Work out the finished part from the listing and answer in its coordinate system (mm). Coordinates: 2 decimals unless noted, no trailing zeros. Loops run counter-clockwise (first coordinate to the right, second up) from the corner with the lowest first, then second, coordinate; pieces in that order, holes last. Notation, with made-up numbers: (38, 55) -> (92, 55) arc R7 cw to (92, 68) -> close; hole circle Ø6 at (-2.5, 14). An arc over 180 degrees is marked (long way). Answer as CSV lines item,"result".
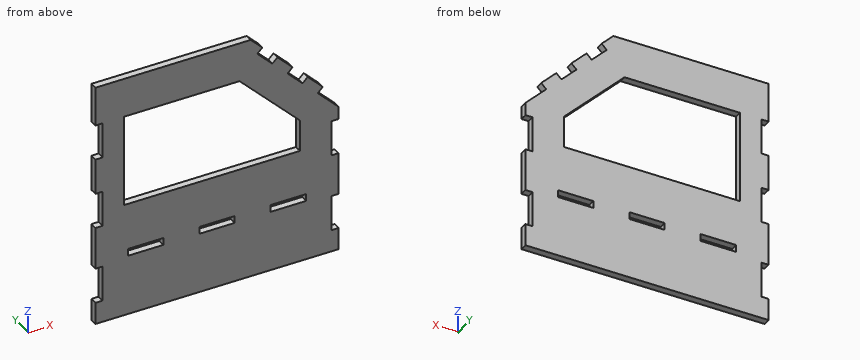
```python
from build123d import *

# Parameters (mm, degrees)
SKETCH_W  = 49.6
SKETCH_H  = 10
PAD_DEPTH = 10


with BuildPart() as part:
    # Sketch → Pad (new body)
    with BuildSketch(Plane.XZ):
        Polygon((0, 0), (0, 30.933), (10, 30.933), (10, 80.733), (0, 80.733), (0, 140.2), (10, 140.2), (10, 190), (0, 190), (0, 240), (10, 240), (10, 289.8), (0, 289.8), (0, 345), (217.0709, 345), (233.405067, 328.665833), (226.333999, 321.594766), (247.405781, 300.522983), (254.476849, 307.594051), (275.690052, 286.380848), (268.618985, 279.30978), (289.690767, 258.237998), (296.761835, 265.309066), (317.975038, 244.095862), (310.90397, 237.024795), (340, 207.928765), (340, 189.999765), (330, 189.999765), (330, 140.199765), (340, 140.199765), (340, 80.733), (330, 80.733), (330, 30.933), (340, 30.933), (340, 0), align=None)
        with Locations((70.2, 90)):
            Rectangle(SKETCH_W, SKETCH_H, mode=Mode.SUBTRACT)
        with Locations((170, 90)):
            Rectangle(SKETCH_W, SKETCH_H, mode=Mode.SUBTRACT)
        with Locations((269.8, 90)):
            Rectangle(SKETCH_W, SKETCH_H, mode=Mode.SUBTRACT)
        Polygon((40, 289.8), (40, 160.8), (286, 160.8), (286, 205.3), (201.5, 289.8), align=None, mode=Mode.SUBTRACT)
    extrude(amount=PAD_DEPTH)


solid = part.part
```
(1) A cutting plane is placed at A-A, the plane x = 208.5. Write down the section's boundary in (y, z).
Computed values:
outline,"(-10, 0) -> (0, 0) -> (0, 160.8) -> (-10, 160.8) -> close; (-10, 282.8) -> (0, 282.8) -> (0, 345) -> (-10, 345) -> close"
(2) A cutting plane is placed at B-B, the plane z = 183. Write down the section's boundary in (x, y), and give its area (3 significant figures).
Computed values:
outline,"(10, -10) -> (40, -10) -> (40, 0) -> (10, 0) -> close; (286, -10) -> (330, -10) -> (330, 0) -> (286, 0) -> close"
area,"740 mm2"
(3) Flat-ended cylindrical pins translate along their axes: pin 1 Ø5 at (y, z) = (-6.5, 87.5) entering from -X; pin 2 Ø5 at (y, z) = (-4, 53) entering from +X; pin 3 Ø3 at (y, z) = (-4.5, 179.5) entering from -X; pin 4 Ø5 at (x, y) = (334, -5.5) entering from +Z. Find the tip coordinate at first contact, or state that the pin passes through.
Computed values:
pin 1,"x = 0"
pin 2,"x = 330"
pin 3,"x = 10"
pin 4,"z = 216.43"
(4) Consider line 1 along Z through (x, y) = (181, -6.5); line 2 along X through (y, z) = (-3.25, 88.5); line 3 along Z through (x, y) = (261, -2.25). Determine where each line is inside the solid, lowest interval first.
Computed values:
line 1,"0 to 85, 95 to 160.8, 289.8 to 345"
line 2,"0 to 45.4, 95 to 145.2, 194.8 to 245, 294.6 to 340"
line 3,"0 to 85, 95 to 160.8, 230.3 to 301.07"
(5) A cutting plane is placed at C-C, the plane x = 151. Write down the section's boundary in (y, z), and give its area (3 significant figures).
Computed values:
outline,"(-10, 0) -> (0, 0) -> (0, 85) -> (-10, 85) -> close; (-10, 95) -> (0, 95) -> (0, 160.8) -> (-10, 160.8) -> close; (-10, 289.8) -> (0, 289.8) -> (0, 345) -> (-10, 345) -> close"
area,"2,060 mm2"
(6) A cutting plane is placed at D-D, the plane y = -2.5. Count the separate pieces of the cut face and the enclosed holes in it, and give its area (3 significant figures).
Computed values:
separate pieces,"1"
enclosed holes,"4"
area,"76,600 mm2"
